For this review, take the finished solid that the model builds, in its own axes (mm). Face numbers are marked on the shaded views. A direction names the side the tool comes from. Give positions to 0.01 mm unless a question says otherwise; leave off trailing zeros. Order: outer loops, then holes, each group sorted by start corner. A loop starts at its lowest first (then second) coordinate and runs counter-clockwise, first axis right, second up. Notation, with made-up numbers: M 15.25,46 L 40.25,46 A28 ccw 40.25,70 Z; hole C 80.5,-25 d1. An arc over 180 degrees is marked long. Use CSV: the item, a comma, the result in double quotes. Start each with the question number.
(1) Draft analysis for pull direction Z (two halves, no side actions). For the marked faces 1, 2 and 3, state which applies: pulls with the +Z half, pulls with the -Z half, needs draft (parallel to the pull), parting line crosses it, or undercut.
(2) Consider section B-B (y = 33.5). Write out the cut boundary in (x, z).
(3) Consider section A-A (y = 17.5). Write out the cut boundary in (x, z), and give its area (3 significant figures).
(4) Wall thickness on L1, parallel to Z at x = 0, y = 29; L2, parallel to X at y = 7.5, z = 3.25; L3, parallel to Z at x = 3.75, y = 7: over which ranges is each line inside the solid? List them lowest first. Write a range as from..to.
(5) Tool access review of the marked faces 4, 5 and 6: name each direction out of +Z, -Z, +X, -X, +Y, -Y from which nothing blocks a thin tool from reaching the whole face with its end or side.
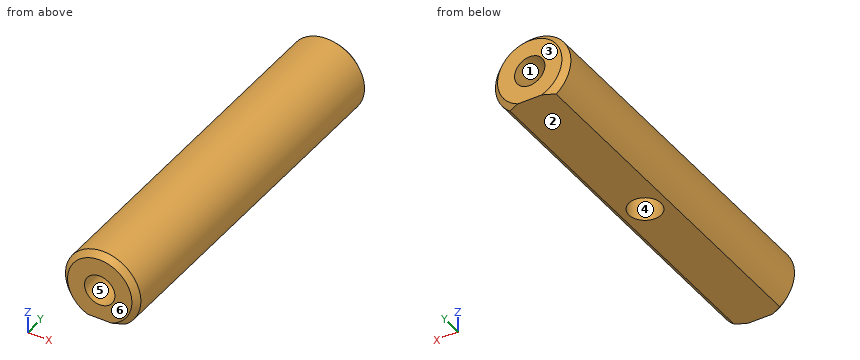
```python
from build123d import *
from OCP.BRepAlgoAPI import BRepAlgoAPI_Cut
from OCP.TopTools import TopTools_ListOfShape

# Parameters (mm, degrees)
BOSS_EXTRUDE2_DEPTH       = 40
CUT_EXTRUDE1_START        = -7.349615
SKETCH2_R                 = 1.75
CUT_EXTRUDE1_DEPTH        = 4
F_1_0MM_DOWEL_HOLE1_D     = 3.3
F_1_0MM_DOWEL_HOLE1_DEPTH = 14.008579979
F_1_0MM_DOWEL_HOLE1_TIP   = 0.991420021
F_1_0MM_DOWEL_HOLE2_D     = 3.3
F_1_0MM_DOWEL_HOLE2_DEPTH = 14.008579979
F_1_0MM_DOWEL_HOLE2_TIP   = 0.991420021
CHAMFER1_SIZE             = 0.6
CHAMFER2_SIZE             = 0.6


with BuildPart() as part:
    # Sketch1 → Boss-Extrude2 (new body)
    with BuildSketch(Plane(origin=(0, 0, 0), x_dir=(1, 0, 0), z_dir=(0, 1, 0))):
        with BuildLine():
            Line((2.5, 3.249615362), (-2.5, 3.249615362))
            ThreePointArc((-2.5, 3.249615362), (0, -4.1), (2.5, 3.249615362))
        make_face()
    extrude(amount=BOSS_EXTRUDE2_DEPTH)


with BuildPart() as cut_extrude1_tool:
    # Sketch2 → Cut-Extrude1 (new body)
    with BuildSketch(Plane.XY.offset(4.1).offset(CUT_EXTRUDE1_START)):
        with Locations(Location((0, 20, 0), (0, 0, 180))):
            Circle(SKETCH2_R)
    extrude(amount=CUT_EXTRUDE1_DEPTH)


with BuildPart() as part_1:
    add(part.part)

    # Cut-Extrude1: cut by cut_extrude1_tool, with a tolerance
    cut_extrude1_stock = TopTools_ListOfShape()
    cut_extrude1_stock.Append(part_1.part.wrapped)
    cut_extrude1_tools = TopTools_ListOfShape()
    cut_extrude1_tools.Append(cut_extrude1_tool.part.wrapped)
    cut_extrude1_cut = BRepAlgoAPI_Cut()
    cut_extrude1_cut.SetArguments(cut_extrude1_stock)
    cut_extrude1_cut.SetTools(cut_extrude1_tools)
    cut_extrude1_cut.SetFuzzyValue(0.00001)
    cut_extrude1_cut.Build()
    add(Compound.cast(cut_extrude1_cut.Shape()).solids(), mode=Mode.REPLACE)

    # Ø1.0mm Dowel Hole1
    with Locations(Plane(origin=(0, 40, 0), x_dir=(1, 0, 0), z_dir=(0, 1, 0))):
        with Locations((0, 0)):
            Hole(F_1_0MM_DOWEL_HOLE1_D / 2, depth=F_1_0MM_DOWEL_HOLE1_DEPTH)
            with Locations((0, 0, -(F_1_0MM_DOWEL_HOLE1_DEPTH + F_1_0MM_DOWEL_HOLE1_TIP / 2))):  # 118° drill point
                Cone(0, F_1_0MM_DOWEL_HOLE1_D / 2, F_1_0MM_DOWEL_HOLE1_TIP, mode=Mode.SUBTRACT)

    # Ø1.0mm Dowel Hole2
    with Locations(Plane(origin=(0, 0, 0), x_dir=(-1, 0, 0), z_dir=(0, -1, 0))):
        with Locations((0, 0)):
            Hole(F_1_0MM_DOWEL_HOLE2_D / 2, depth=F_1_0MM_DOWEL_HOLE2_DEPTH)
            with Locations((0, 0, -(F_1_0MM_DOWEL_HOLE2_DEPTH + F_1_0MM_DOWEL_HOLE2_TIP / 2))):  # 118° drill point
                Cone(0, F_1_0MM_DOWEL_HOLE2_D / 2, F_1_0MM_DOWEL_HOLE2_TIP, mode=Mode.SUBTRACT)

    # Chamfer1
    chamfer1_edges = [part_1.edges().sort_by_distance(p)[0] for p in [
        (0, 40, 4.1),
    ]]
    chamfer(chamfer1_edges, length=CHAMFER1_SIZE)

    # Chamfer2
    chamfer2_edges = [part_1.edges().sort_by_distance(p)[0] for p in [
        (0, 0, 4.1),
    ]]
    chamfer(chamfer2_edges, length=CHAMFER2_SIZE)


solid = part_1.part
```
Check result:
1,face 1,"undercut"
1,face 2,"pulls with the -Z half"
1,face 3,"needs draft"
2,outline,"M -2.5,-3.25 L 2.5,-3.25 A4.1 ccw long Z; hole C 0,0 d3.3"
3,outline,"M -2.5,-3.25 L 2.5,-3.25 A4.1 ccw long Z"
3,area,"49.9 mm^2"
4,L1,"z = -3.25..-1.65, 1.65..4.1"
4,L2,"x = -2.5..2.5"
4,L3,"z = -1.66..1.66"
5,face 4,"-Z"
5,face 5,"-Y"
5,face 6,"+Z, -Z, +X, -X, -Y"
